```python
from build123d import *

# Parameters (mm, degrees)
BOSS_EXTRUDE1_DEPTH        = 12.7
M8X1_25_TAPPED_HOLE1_D     = 6.8
M8X1_25_TAPPED_HOLE1_DEPTH = 9.147932364
M8X1_25_TAPPED_HOLE1_TIP   = 2.042926105
M8X1_25_TAPPED_HOLE2_D     = 6.8
M8X1_25_TAPPED_HOLE2_DEPTH = 9.147932364
M8X1_25_TAPPED_HOLE2_TIP   = 2.042926105
FILLET3_R                  = 2.5
FILLET5_R                  = 2.5
FILLET6_R                  = 2.5
FILLET7_R                  = 2.5


with BuildPart() as part:
    # Sketch1 → Boss-Extrude1 (new body)
    with BuildSketch(Plane.XY):
        Polygon((25.5, 32), (25.5, 19.738981448), (-6.106181157, 19.738981448), (-6.106181157, 10.852067636), (25.5, 10.852067636), (25.5, -32), (-25.5, -32), (-25.5, -19.738981448), (6.242414697, -19.738981448), (6.242414697, -10.852067636), (-25.5, -10.852067636), (-25.5, 32), align=None)
    extrude(amount=BOSS_EXTRUDE1_DEPTH)

    # M8x1.25 Tapped Hole1
    with Locations(Plane(origin=(0, 32, 0), x_dir=(1, 0, 0), z_dir=(0, 1, 0))):
        with Locations((0, -6.35)):
            Hole(M8X1_25_TAPPED_HOLE1_D / 2, depth=M8X1_25_TAPPED_HOLE1_DEPTH)
            with Locations((0, 0, -(M8X1_25_TAPPED_HOLE1_DEPTH + M8X1_25_TAPPED_HOLE1_TIP / 2))):  # 118° drill point
                Cone(0, M8X1_25_TAPPED_HOLE1_D / 2, M8X1_25_TAPPED_HOLE1_TIP, mode=Mode.SUBTRACT)

    # M8x1.25 Tapped Hole2
    with Locations(Plane(origin=(0, -32, 0), x_dir=(-1, 0, 0), z_dir=(0, -1, 0))):
        with Locations((0, -6.35)):
            Hole(M8X1_25_TAPPED_HOLE2_D / 2, depth=M8X1_25_TAPPED_HOLE2_DEPTH)
            with Locations((0, 0, -(M8X1_25_TAPPED_HOLE2_DEPTH + M8X1_25_TAPPED_HOLE2_TIP / 2))):  # 118° drill point
                Cone(0, M8X1_25_TAPPED_HOLE2_D / 2, M8X1_25_TAPPED_HOLE2_TIP, mode=Mode.SUBTRACT)

    # Fillet3
    fillet3_edges = [part.edges().sort_by_distance(p)[0] for p in [
        (-6.106181157, 19.738981448, 6.35),
    ]]
    fillet(fillet3_edges, radius=FILLET3_R)

    # Fillet5
    fillet5_edges = [part.edges().sort_by_distance(p)[0] for p in [
        (-6.106181157, 10.852067636, 6.35),
    ]]
    fillet(fillet5_edges, radius=FILLET5_R)

    # Fillet6
    fillet6_edges = [part.edges().sort_by_distance(p)[0] for p in [
        (6.242414697, -10.852067636, 6.35),
    ]]
    fillet(fillet6_edges, radius=FILLET6_R)

    # Fillet7
    fillet7_edges = [part.edges().sort_by_distance(p)[0] for p in [
        (6.242414697, -19.738981448, 6.35),
    ]]
    fillet(fillet7_edges, radius=FILLET7_R)


solid = part.part
```
Design review of the part built by this model. Coordinates are the model's own, in mm. A direction names the side the tool comes from. Round coordinates to 2 decimals unless told otherwise and drop trailing zeros. Write each loop counter-clockwise with the first axis right and the second up, starting at its lowest first coordinate (ties: lowest second). Pieces come first, ordered by that corner, then holes. Notation, with made-up numbers: (58.5, -5) -> (78.5, -5) arc R13 cw to (78.5, 6) -> close; hole circle Ø8 at (14.5, 46.25). An arc over 180 degrees is marked (long way). Write item = value, one per line. Start each with the question number.
1) Clearance check with flat-ended pins moving along their axes: pin 1 (1.9 mm diameter, centred on y = 15.5, z = 9.5, fed in from +X); pin 2 (4 mm diameter, centred on x = -5, y = -18.5, fed in from +Z); pin 3 (1.9 mm diameter, centred on y = -15, z = 8, fed in from -X). State where each tip first meets the part, or that it passes through.
2) Take a section at D-D, the plane y = -14.5. State the section outline as (x, z) points, plus the area to 3 significant figures.
3) Tool access review of faces 4 (the face through (0, -32, 10)), 5 (the face through (-5.35, 19.03, 6.44)), 6 (the face through (25.5, -10, 6)), 7 (the face through (0.74, 27.36, 9.67)), 8 (the face through (5.53, -18.987, 6.439)): name each direction out of +Z, -Z, +X, -X, +Y, -Y from which nothing blocks a thin tool from reaching the whole face with its end or side.
4) Mouldability with a two-part tool opening along X and no side actions: class faces 1 (the face through (-5.39, 11.6, 6.44)), 2 (the face through (-0.74, -27.36, 9.67)), 3 (the face through (-25.5, 10, 6)) as +X half, -X half, draft (parallel to the pull), parting line (faces both ways), or undercut.
5) Take a section at B-B, the plane x = -13.5. State the section outline as (y, z) points, plus the area to 3 significant figures.
6) Wall thickness on probe 1 along Y at (x, z) = (1.5, 9.5); probe 2 along Y at (x, z) = (-16, 2); probe 3 along Y at (x, z) = (2, 9): over which ranges is each line inside the solid? List them lowest first. Write a range as from..to.
7) Take a section at A-A, the plane z = 10.5. State the section outline as (x, y) points, plus the area to 3 significant figures.
8) Take a section at C-C, the plane y = 27. State the section outline as (x, z) points.
Results list:
q1.pin_1 = -6.11
q1.pin_2 = 12.7
q1.pin_3 = 6.24
q2.outline = (6.24, 0) -> (25.5, 0) -> (25.5, 12.7) -> (6.24, 12.7) -> close
q2.area = 245 mm²
q3.face_4 = +Z, -Z, +X, -X, -Y
q3.face_5 = +Z, -Z, +X
q3.face_6 = +Z, -Z, +X, +Y, -Y
q3.face_7 = +Y
q3.face_8 = +Z, -Z, -X
q4.face_1 = +X half
q4.face_2 = undercut
q4.face_3 = -X half
q5.outline = (-32, 0) -> (-19.74, 0) -> (-19.74, 12.7) -> (-32, 12.7) -> close; (-10.85, 0) -> (32, 0) -> (32, 12.7) -> (-10.85, 12.7) -> close
q5.area = 700 mm²
q6.probe_1 = -32..-19.74, -10.85..10.85, 19.74..32
q6.probe_2 = -32..-19.74, -10.85..32
q6.probe_3 = -22.8..-19.74, -10.85..10.85, 19.74..22.8
q7.outline = (-25.5, -32) -> (25.5, -32) -> (25.5, 10.85) -> (-3.61, 10.85) arc R2.5 cw to (-6.11, 13.35) -> (-6.11, 17.24) arc R2.5 cw to (-3.61, 19.74) -> (25.5, 19.74) -> (25.5, 32) -> (-25.5, 32) -> (-25.5, -10.85) -> (3.74, -10.85) arc R2.5 cw to (6.24, -13.35) -> (6.24, -17.24) arc R2.5 cw to (3.74, -19.74) -> (-25.5, -19.74) -> close
q7.area = 2,710 mm²
q8.outline = (-25.5, 0) -> (25.5, 0) -> (25.5, 12.7) -> (-25.5, 12.7) -> close; hole circle Ø6.8 at (0, 6.35)
